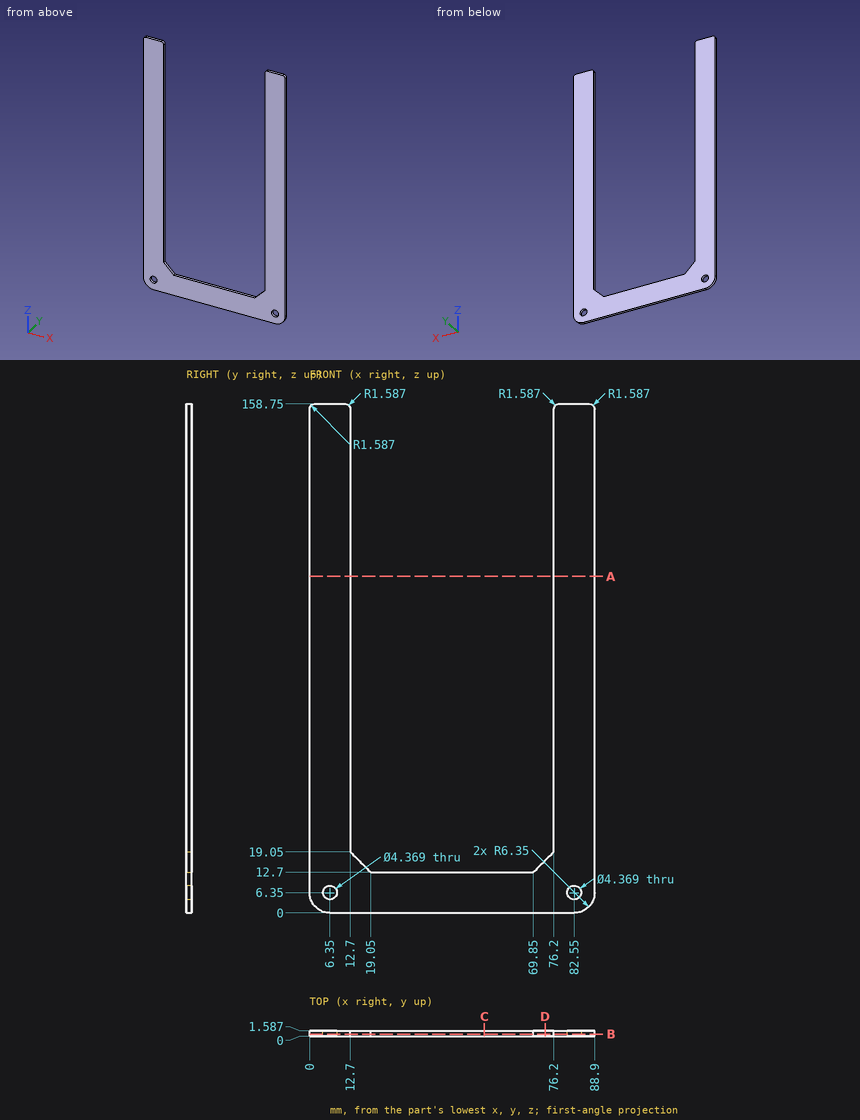
The figure shows three views and two pictorial views of one solid part (mm, origin at its lowest corner). Answer the questions. Round coordinates to 2 decimals unless told otherwise and drop trailing zeros. Order: outer loops, then holes, each group sorted by start corner. A loop starts at its lowest first (then second) coordinate and runs counter-clockwise, first axis right, second up. Notation, with made-up numbers: (-30.5, 3.5) -> (21.5, 3.5) arc R16 ccw to (21.5, 13.5) -> close; hole circle Ø5 at (29.5, 63.25). An arc over 180 degrees is marked (long way). One line per item, written item: value.
Item 1: Straight lines are drawn through the part: L1, parallel to X at y = 0.5, z = 142; L2, parallel to Z at x = 82.5, y = 0.3; L3, parallel to X at y = 1.15, z = 7 (1 decimal). For each, find the intervals that lie inside material, in ascending order.
Taken from the geometry:
L1: x = 0 to 12.7, 76.2 to 88.9
L2: z = 0 to 4.17, 8.53 to 158.75
L3: x = 0 to 4.3, 8.4 to 80.5, 84.6 to 88.9
Item 2: Find section D-D, the plane x = 73.5. Give the vertices of the cut face in (y, z).
Taken from the geometry:
outline: (0, 0) -> (1.59, 0) -> (1.59, 16.35) -> (0, 16.35) -> close
Item 3: Find section B-B, the plane y = 0.55. State how many separate pieces and enclosed holes the cut face has, then the cut area to 3 significant figures.
Taken from the geometry:
separate pieces: 1
enclosed holes: 2
area: 4,830 mm2
Item 4: Find section A-A, the plane z = 105. Give the vertices of the cut face in (x, y).
Taken from the geometry:
outline: (0, 0) -> (12.7, 0) -> (12.7, 1.59) -> (0, 1.59) -> close; (76.2, 0) -> (88.9, 0) -> (88.9, 1.59) -> (76.2, 1.59) -> close
Item 5: Find section C-C, the plane x = 54.5. Give the vertices of the cut face in (y, z).
Taken from the geometry:
outline: (0, 0) -> (1.59, 0) -> (1.59, 12.7) -> (0, 12.7) -> close
